Part model, mm, in its own coordinate system. Face numbers are marked on the shaded views. A direction names the side the tool comes from. Round coordinates to 2 decimals unless told otherwise and drop trailing zeros. Write each loop counter-clockwise with the first axis right and the second up, starting at its lowest first coordinate (ties: lowest second). Pieces come first, ordered by that corner, then holes.
1) Which spindle directions (+Z, -Z, +X, -X, +Y, -Y) get a long thin tool onto all of the face, cutting with end or side? Do the marked faces 1, 2 and 3. Say none if no direction does.
2) Saw through at C-C on z = 2.25. Write the cut outline in (x, y) (3 decimals), and give its area (3 significant figures).
3) Saw through at A-A on y = 17. Write the cut outline in (x, z) (3 decimals), and give its area (3 significant figures).
4) Saw through at D-D on x = 7.25. Write the cut outline in (y, z) (3 decimals).
5) Flat gauge pins, fed straight in: pin 1 (3.5 mm diameter, centred on y = 18, z = -4, fed in from +X); pin 2 (0.7 mm diameter, centred on x = 0.5, z = -6, fed in from -Y) (3 decimals); pin 3 (1 mm diameter, centred on x = 2.5, y = -9, fed in from -Z). Where does each tip first touch, or does it go through?
6) Drill centre lines: L1, parallel to Z at x = -6, y = 7; L2, parallel to Y at x = -5.25, z = 3.75 (3 decimals); L3, parallel to Y at x = 0.5, z = -6 (3 decimals). Where is each one in solid material? Low to high.
7) Saw through at B-B on y = -7. Write the cut outline in (x, z) (3 decimals), and give its area (3 significant figures).
```python
from build123d import *

# Parameters (mm, degrees)
F0_W     = 23.45
F0_H     = 42.01
F1_DEPTH = 5.63
F2_T     = -1
F3_W     = 4
F3_H     = 6.987
F4_DEPTH = 2.2
F5_W     = 4
F5_H     = 1.456921
F6_DEPTH = 9


with BuildPart() as f1:
    # F0 (on Top) → F1 (new body)
    with BuildSketch(Plane.XY):
        Rectangle(F0_W, F0_H)
    extrude(amount=F1_DEPTH)

    # F2
    f2_openings = [f1.faces().sort_by_distance(p)[0] for p in [
        (0, 21.005, 2.815),
    ]]
    offset(amount=F2_T, openings=f2_openings)

    # F3 (on face) → F4 (join)
    with BuildSketch(Plane(origin=(0, 21.005, 0), x_dir=(-1, 0, 0), z_dir=(0, 1, 0))):
        with Locations((-0.08324, -3.4935)):
            Rectangle(F3_W, F3_H)
    extrude(amount=-F4_DEPTH)

    # F5 (on face) → F6 (join)
    with BuildSketch(Plane.XZ.offset(-18.805)):
        with Locations((0.08324, -6.258539)):
            Rectangle(F5_W, F5_H)
    extrude(amount=F6_DEPTH)


solid = f1.part
```
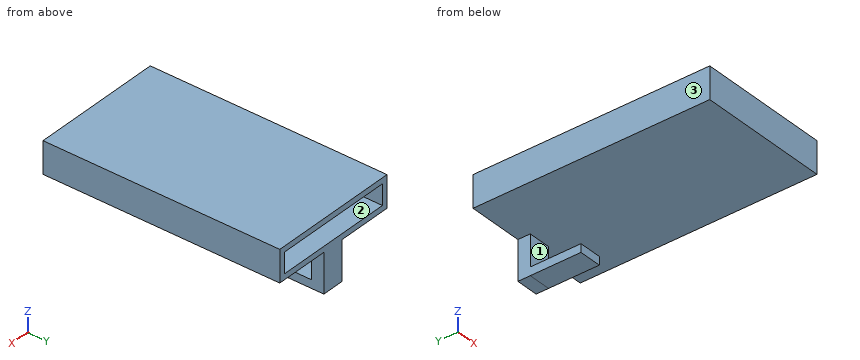
Completed:
1. face 1: +X, -X, -Y
1. face 2: +Y
1. face 3: +Z, -Z, -X, +Y, -Y
2. outline: (-11.725, -21.005) - (11.725, -21.005) - (11.725, 21.005) - (10.725, 21.005) - (10.725, -20.005) - (-10.725, -20.005) - (-10.725, 21.005) - (-11.725, 21.005) - close
2. area: 105 mm2
3. outline: (-11.725, 0) - (11.725, 0) - (11.725, 5.63) - (-11.725, 5.63) - close; (-1.917, -6.987) - (2.083, -6.987) - (2.083, -5.53) - (-1.917, -5.53) - close; hole (-10.725, 1) - (10.725, 1) - (10.725, 4.63) - (-10.725, 4.63) - close
3. area: 60.0 mm2
4. outline: (-21.005, 0) - (21.005, 0) - (21.005, 1) - (-20.005, 1) - (-20.005, 4.63) - (21.005, 4.63) - (21.005, 5.63) - (-21.005, 5.63) - close
5. pin 1: stops at x = 2.08
5. pin 2: stops at y = 9.805
5. pin 3: stops at z = 0
6. L1: z = 0 to 1, 4.63 to 5.63
6. L2: y = -21.005 to -20.005
6. L3: y = 9.805 to 21.005
7. outline: (-11.725, 0) - (11.725, 0) - (11.725, 5.63) - (-11.725, 5.63) - close; hole (-10.725, 1) - (10.725, 1) - (10.725, 4.63) - (-10.725, 4.63) - close
7. area: 54.2 mm2
